from build123d import *

# Parameters (mm, degrees)
F1_DEPTH = 95.25
F0_R     = 11.1125
F2_DEPTH = 11.1125
F3_R     = 11.1125
F4_DEPTH = 11.1125
F5_R     = 19.05


with BuildPart() as f1:
    # F0 (on Front) → F1 (new body)
    with BuildSketch(Plane.XZ):
        with BuildLine():
            Line((31.75, 0), (42.8625, 0))
            ThreePointArc((42.8625, 0), (0, 42.8625), (-42.8625, 0))
            Line((-42.8625, 0), (-31.75, 0))
            ThreePointArc((-31.75, 0), (0, 31.75), (31.75, 0))
        make_face()
    extrude(amount=F1_DEPTH)

    # F0 (on Front) → F2 (join)
    with BuildSketch(Plane.XZ):
        with BuildLine():
            ThreePointArc((-42.8625, 0), (0, 42.8625), (42.8625, 0))
            Line((42.8625, 0), (57.15, 0))
            Line((57.15, 0), (57.15, 69.85))
            Line((57.15, 69.85), (-57.15, 69.85))
            Line((-57.15, 69.85), (-57.15, 0))
            Line((-57.15, 0), (-42.8625, 0))
        make_face()
        with Locations((-38.1, 50.8)):
            Circle(F0_R, mode=Mode.SUBTRACT)
        with Locations((38.1, 50.8)):
            Circle(F0_R, mode=Mode.SUBTRACT)
    extrude(amount=F2_DEPTH)

    # F3 (on face) → F4 (join)
    with BuildSketch(Plane.XZ.offset(95.25)):
        with BuildLine():
            ThreePointArc((-42.8625, 0), (0, 42.8625), (42.8625, 0))
            Line((42.8625, 0), (57.15, 0))
            Line((57.15, 0), (57.15, 69.85))
            Line((57.15, 69.85), (-57.15, 69.85))
            Line((-57.15, 69.85), (-57.15, 0))
            Line((-57.15, 0), (-42.8625, 0))
        make_face()
        with Locations((-38.1, 50.8)):
            Circle(F3_R, mode=Mode.SUBTRACT)
        with Locations((38.1, 50.8)):
            Circle(F3_R, mode=Mode.SUBTRACT)
    extrude(amount=-F4_DEPTH)

    # F5
    f5_edges = [f1.edges().sort_by_distance(p)[0] for p in [
        (57.15, -89.69375, 69.85),
        (-57.15, -5.55625, 69.85),
        (-57.15, -89.69375, 69.85),
        (57.15, -5.55625, 69.85),
    ]]
    fillet(f5_edges, radius=F5_R)


solid = f1.part
Source: CAD feature listing. Evaluate the final solid. Frame: model axes, mm. A direction names the side the tool comes from. Give positions to 0.01 mm unless a question says otherwise; leave off trailing zeros. Order: outer loops, then holes, each group sorted by start corner. A loop starts at its lowest first (then second) coordinate and runs counter-clockwise, first axis right, second up. Notation, with made-up numbers: (0.25, 71) -> (19.25, 71) arc R18 cw to (19.25, 93) -> close; hole circle Ø10 at (16, -19.5). An arc over 180 degrees is marked (long way). Use a Markdown table: item, result.
1) Section query D-D, the plane x = -23.5. Return the cut outline in (y, z), then the cut area to 3 significant figures.
Answer list:
| item | result |
|---|---|
| outline | (-95.25, 21.35) -> (0, 21.35) -> (0, 69.85) -> (-11.11, 69.85) -> (-11.11, 35.85) -> (-84.14, 35.85) -> (-84.14, 69.85) -> (-95.25, 69.85) -> close |
| area | 2,140 mm² |
2) Ray query, line 1 along X through (y, z) = (-4, 50); line 2 along Z through (x, y) = (-38.1, -88); line 3 along Y through (x, z) = (-5.5, 51). Return the intervals inside material, ascending. Write a range as [from, to].
Answer list:
| item | result |
|---|---|
| line 1 | [-57.15, -49.18], [-27.02, 27.02], [49.18, 57.15] |
| line 2 | [0, 39.69], [61.91, 69.85] |
| line 3 | [-95.25, -84.14], [-11.11, 0] |
3) Section query A-A, the plane z = 45. Return the cut outline in (x, y), then the cut area to 3 significant figures.
Answer list:
| item | result |
|---|---|
| outline | (-57.15, -95.25) -> (-47.58, -95.25) -> (-47.58, -84.14) -> (-57.15, -84.14) -> close; (-57.15, -11.11) -> (-47.58, -11.11) -> (-47.58, 0) -> (-57.15, 0) -> close; (-28.62, -95.25) -> (28.62, -95.25) -> (28.62, -84.14) -> (-28.62, -84.14) -> close; (-28.62, -11.11) -> (28.62, -11.11) -> (28.62, 0) -> (-28.62, 0) -> close; (47.58, -95.25) -> (57.15, -95.25) -> (57.15, -84.14) -> (47.58, -84.14) -> close; (47.58, -11.11) -> (57.15, -11.11) -> (57.15, 0) -> (47.58, 0) -> close |
| area | 1,700 mm² |
4) Reachability of faces 5 (the cylindrical face through (0.943, -47.114, 42.852)), 6 (the flat face through (-57.15, -90, 26)) from +Z, -Z, +X, -X, +Y, -Y: full face, straight path, thin tool, end or side. Return the list, or none.
Answer list:
| item | result |
|---|---|
| face 5 | +Z |
| face 6 | +Z, -Z, -X, +Y, -Y |
5) Section query C-C, the plane z = 28. Return the cut outline in (x, y).
Answer list:
| item | result |
|---|---|
| outline | (-57.15, -95.25) -> (-14.97, -95.25) -> (-14.97, 0) -> (-57.15, 0) -> (-57.15, -11.11) -> (-32.45, -11.11) -> (-32.45, -84.14) -> (-57.15, -84.14) -> close; (14.97, -95.25) -> (57.15, -95.25) -> (57.15, -84.14) -> (32.45, -84.14) -> (32.45, -11.11) -> (57.15, -11.11) -> (57.15, 0) -> (14.97, 0) -> close |
6) Section query B-B, the plane x = 36. Return the cut outline in (y, z).
Answer list:
| item | result |
|---|---|
| outline | (-95.25, 0) -> (0, 0) -> (0, 39.89) -> (-11.11, 39.89) -> (-11.11, 23.26) -> (-84.14, 23.26) -> (-84.14, 39.89) -> (-95.25, 39.89) -> close; (-95.25, 61.71) -> (-84.14, 61.71) -> (-84.14, 69.85) -> (-95.25, 69.85) -> close; (-11.11, 61.71) -> (0, 61.71) -> (0, 69.85) -> (-11.11, 69.85) -> close |
7) Mould query, pull axis Y, two halves, no side actions, for faces 1 (the flat face through (-1, -95.25, 35)), 2 (the flat face through (-0.8, -11.112, 43.2)), 3 (the cylindrical face through (-51.42, -5.63, 64.42)), 4 (the flat face through (-1, 0, 35)). Classes: +Y half, -Y half, draft (parallel to the pull), parting line (faces both ways), or undercut.
Answer list:
| item | result |
|---|---|
| face 1 | -Y half |
| face 2 | undercut |
| face 3 | draft |
| face 4 | +Y half |
8) Contact query for flat-ended pins moving along their axis: P1, Ø2, axis at y = -68, z = 38, coming from the +X side; P2, Ø1.5, axis at y = -56, z = 20.5, coming from the -X side; P3, Ø6, axis at x = -20.5, y = -82, coming from the -Z side. Output: stop coordinate, or through.
Answer list:
| item | result |
|---|---|
| P1 | x = 21.64 |
| P2 | x = -38.04 |
| P3 | z = 21.35 |
